The listing builds one solid part. Answer for the finished solid, in the listing's coordinates (mm). Coordinates: 2 decimals unless noted, no trailing zeros. Order: outer loops, then holes, each group sorted by start corner. A loop starts at its lowest first (then second) coordinate and runs counter-clockwise, first axis right, second up.
Autodesk Inventor part; units mm, degrees
ref_plane "YZ Plane" through (0, 0, 0) normal (1, 0, 0) x (0, 1, 0)
ref_plane "XZ Plane" through (0, 0, 0) normal (0, 1, 0) x (-1, 0, 0)
ref_plane "XY Plane" through (0, 0, 0) normal (0, 0, 1) x (1, 0, 0)
sketch "Эскиз1" plane through (0, 0, 0) normal (0, 0, 1) x (1, 0, 0)
  line L0 (-13, 0) -> (13, 0)
  line L1 (-47.5, 180) -> (47.5, 180)
  line L2 (-16.5, 130) -> (16.5, 130)
  line L3 (-12.9827, 110) -> (12.9827, 110)
  line L4 (-11.8003, 90) -> (11.8003, 90)
  line L5 (47.5, 180) -> (37.594, 168.7363)
  line L6 (-47.5, 180) -> (-37.594, 168.7363)
  line L7 (-37.594, 168.7363) -> (37.594, 168.7363)
  arc A0 (37.594, 168.7363) -> (12.9827, 110) centre (112.573, 102.7948) ccw
  arc A1 (12.9827, 110) -> (13, 0) centre (771.5375, 55.1194) ccw
  arc A2 (-12.9827, 110) -> (-37.594, 168.7363) centre (-112.573, 102.7948) ccw
  arc A3 (-13, 0) -> (-12.9827, 110) centre (-771.5375, 55.1194) ccw
  line L8 (-11, 80.4723) -> (-11, 26.1046)
  line L9 (11, 80.4723) -> (11, 26.1046)
  line L10 (-37.594, 168.7363) -> (13.0707, 111.1279)
  line L11 (37.594, 168.7363) -> (-13.0707, 111.1279)
  point P0 (0, 0)
  point P1 (0, 0)
  point P2 (0, 180)
  point P3 (0, 130)
  point P4 (0, 90)
  point P5 (0, 110)
  point P6 (-11, 55.1194)
  dimension "d0" = 26
  dimension "d1" = 95
  dimension "d2" = 33
  dimension "d5" = 180
  dimension "d6" = 50
  dimension "d7" = 20
  dimension "d8" = 20
  dimension "d9" = 15
  dimension "d10" = 15
  dimension "d13" = 22
  dimension "d19" = 55.1194
extrude "Выдавливание1" add sketch "Эскиз1" along normal blind 25
sketch "Эскиз2" plane through (0, 0, 0) normal (1, 0, 0) x (0, 1, 0)
  line L0 (0, 0) -> (110, 0)
  line L1 (110, 0) -> (110, 25)
  line L2 (0, 25) -> (110, 25)
  line L3 (0, 0) -> (0, 25)
  line L4 (110, 0) -> (169.3956, 0)
  line L5 (110, 25) -> (169.3956, 25)
  line L6 (110, 0) -> (110, 25)
  line L7 (130, 18) -> (130, 7)
  line L8 (55, 21) -> (55, 4)
  arc A0 (0, 25) -> (130, 18) centre (172.2556, 2013.3889) ccw
  arc A1 (130, 7) -> (0, 0) centre (172.2556, -1988.3889) ccw
  line L9 (180, 13) -> (180, 12)
  line L10 (156.0464, 14.5) -> (156.0464, 10.5)
  line L11 (180, 13) -> (156.0464, 14.5)
  line L12 (180, 12) -> (156.0464, 10.5)
  arc A2 (130, 18) -> (156.0464, 14.5) centre (167.6171, 199.2737) ccw
  arc A3 (156.0464, 10.5) -> (130, 7) centre (167.6171, -174.2737) ccw
  line L13 (168.7363, 0) -> (180, 0)
  line L14 (180, 0) -> (180, 25)
  line L15 (168.7363, 25) -> (180, 25)
  point P0 (130, 12.5)
  point P1 (0, 12.5)
  point P2 (55, 12.5)
  point P3 (180, 12.5)
  point P4 (169.3956, 12.5)
  point P5 (156.0464, 12.5)
  point P6 (180, 12.5)
  dimension "d16" = 11
  dimension "d20" = 55
  dimension "d21" = 17
  dimension "d22" = 1
  dimension "d23" = 4
  dimension "d28" = 50
  dimension "d30" = 23.9536
extrude "Выдавливание2" cut sketch "Эскиз2" along normal mid plane 100 contours L3 A0 L8 A1 | L8 A0 L1 A1 | L1 A0 L7 A1 | L7 A2 L10 A3 | L10 L11 L9 L12 keep common part
sketch "Эскиз3" plane through (0, 0, 0) normal (0, 0, 1) x (1, 0, 0)
  arc A0 (37.594, 168.7363) -> (28.1076, 156.0464) centre (112.573, 102.7948) ccw
  line L0 (37.594, 168.7363) -> (47.5, 180)
  line L1 (47.5, 180) -> (-47.5, 180)
  line L2 (-47.5, 180) -> (-37.594, 168.7363)
  arc A1 (-28.1076, 156.0464) -> (-37.594, 168.7363) centre (-112.573, 102.7948) ccw
  line L3 (-28.1076, 156.0464) -> (28.1076, 156.0464)
  line L4 (-28.1076, 156.0464) -> (28.1076, 156.0464)
  line L5 (16.5, 130) -> (-16.5, 130)
  line L6 (16.5, 130) -> (-16.5, 130)
  line L7 (-13, 0) -> (13, 0)
  point P0 (0, 0)
  point P1 (12.9827, 110)
  point P2 (-12.9827, 110)
  point P3 (-30, 158.9361)
  point P4 (30, 158.9361)
  dimension "d31" = 60
  dimension "d32" = 2.8897
properties part number "bachi_v2"
(1) Find section A-A (x = 8.5). Write down the section's boundary in (y, z).
(2) Find section C-C (y = 46). Write down the section's boundary in (x, z), and give its area (3 significant figures).
(3) Find section D-D (x = 21.5). Write down the section's boundary in (y, z).
(4) Each of these flat-tipped pins is pushed along its axis until it touches: pin 1 Ø8 at (x, y) = (-12.5, 53.5) entering from -Z; pin 2 Ø1.5 at (y, z) = (27.5, 6.5) entering from -X; pin 3 Ø12 at (x, y) = (6.5, 53.5) entering from +Z. Where does it stop, or does it pass through?
(5) Consider line 1 (X direction, y = 29.5, z = 15.25); line 2 (Z direction, x = 8, y = 91); line 3 (X direction, y = 66.5, z = 7.5). Determine where each line is inside the solid, lowest interval first.
(6) The mould has two halves that part along Y. Classify faces 1 (the face through (-0.393, 143.144, 15.763)), 2 (the face through (-11.09, 43.54, 12.32)), 3 (the face through (-41.52, 173.2, 12.48)): released by +Y, released by -Y, zero draft, split by the parting line, or undercut.
(7) Find section B-B (z = 2.75). Write down the section's boundary in (x, y), and give its area (3 significant figures).
Findings below:
1. outline: (0, 0) arc R1995.84 cw to (130, 7) arc R185.14 cw to (156.05, 10.5) - (180, 12) - (180, 13) - (156.05, 14.5) arc R185.14 cw to (130, 18) arc R1995.83 cw to (0, 25) - close
2. outline: (-11.05, 3.45) - (11.05, 3.45) - (11.05, 21.55) - (-11.05, 21.55) - close
2. area: 400 mm2
3. outline: (143.73, 9.31) arc R185.14 cw to (156.05, 10.5) - (180, 12) - (180, 13) - (156.05, 14.5) arc R185.14 cw to (143.73, 15.69) - close
4. pin 1: stops at z = 3.69
4. pin 2: stops at x = -11.53
4. pin 3: stops at z = 21.46
5. line 1: x = -11.43 to 11.43
5. line 2: z = 5.79 to 19.21
5. line 3: x = -11.09 to 11.09
6. face 1: released by +Y
6. face 2: undercut
6. face 3: released by -Y
7. outline: (-13, 0) - (13, 0) arc R760.54 cw to (11.26, 35.4) - (-11.26, 35.4) arc R760.53 cw to start
7. area: 849 mm2
